from build123d import *

# Parameters (mm, degrees)
SKETCH1_W                       = 203.2
SKETCH1_H                       = 203.2
BOSS_EXTRUDE1_DEPTH             = 6.35
CUT_EXTRUDE1_REACH              = 8.35
SKETCH2_R                       = 31.75
F_1_4_0_25_DIAMETER_HOLE1_D     = 6.35
F_1_4_0_25_DIAMETER_HOLE1_DEPTH = 6.351
CIRPATTERN1_COUNT               = 12
F_10_32_TAPPED_HOLE1_D          = 4.0386
F_10_32_TAPPED_HOLE1_DEPTH      = 6.351
CIRPATTERN2_COUNT               = 6
CUT_EXTRUDE2_REACH              = 8.35


with BuildPart() as part:
    # Sketch1 → Boss-Extrude1 (new body)
    with BuildSketch(Plane(origin=(0, 0, 0), x_dir=(1, 0, 0), z_dir=(0, 1, 0))):
        Rectangle(SKETCH1_W, SKETCH1_H)
    extrude(amount=BOSS_EXTRUDE1_DEPTH)

    # Sketch2 → Cut-Extrude1 (cut, up to next)
    with BuildSketch(Plane(origin=(0, 6.35, 0), x_dir=(1, 0, 0), z_dir=(0, 1, 0)), mode=Mode.PRIVATE) as cut_extrude1_sk1:
        with Locations(Location((0, 0, 0), (0, 0, 270))):  # turned: the seam where the file's is
            Circle(SKETCH2_R)
    cut_extrude1_tool1 = extrude(cut_extrude1_sk1.sketch, amount=-CUT_EXTRUDE1_REACH, mode=Mode.PRIVATE) & part.part
    add(cut_extrude1_tool1.solids().sort_by_distance((0, 6.35, 0))[0], mode=Mode.SUBTRACT)

    # 1/4 (0.25) Diameter Hole1
    with Locations(Plane(origin=(0, 6.35, 0), x_dir=(1, 0, 0), z_dir=(0, 1, 0))):
        with Locations((0, 85.725)):
            f_1_4_0_25_diameter_hole1 = Hole(F_1_4_0_25_DIAMETER_HOLE1_D / 2, depth=F_1_4_0_25_DIAMETER_HOLE1_DEPTH)

    # CirPattern1: 1/4 (0.25) Diameter Hole1 ×12 about axis
    cirpattern1_axis = Axis((0, 0, 0), (0, 1, 0))
    for i in range(1, CIRPATTERN1_COUNT):
        add(f_1_4_0_25_diameter_hole1.rotate(cirpattern1_axis, i * 360 / CIRPATTERN1_COUNT), mode=Mode.SUBTRACT)

    # #10-32 Tapped Hole1
    with Locations(Plane(origin=(0, 6.35, 0), x_dir=(1, 0, 0), z_dir=(0, 1, 0))):
        with Locations((0, 36.5125)):
            f_10_32_tapped_hole1 = Hole(F_10_32_TAPPED_HOLE1_D / 2, depth=F_10_32_TAPPED_HOLE1_DEPTH)

    # CirPattern2: #10-32 Tapped Hole1 ×6 about axis
    cirpattern2_axis = Axis((0, 0, 0), (0, 1, 0))
    for i in range(1, CIRPATTERN2_COUNT):
        add(f_10_32_tapped_hole1.rotate(cirpattern2_axis, i * 360 / CIRPATTERN2_COUNT), mode=Mode.SUBTRACT)

    # Sketch7 → Cut-Extrude2 (cut, up to next)
    with BuildSketch(Plane(origin=(0, 6.35, 0), x_dir=(1, 0, 0), z_dir=(0, 1, 0)), mode=Mode.PRIVATE) as cut_extrude2_sk1:
        with BuildLine():
            ThreePointArc((96.684914721, 45.084916162), (75.434151417, 75.434151417), (45.084916162, 96.684914721))
            ThreePointArc((45.084916162, 96.684914721), (40.865575958, 95.149200478), (42.4012902, 90.929860273))
            ThreePointArc((42.4012902, 90.929860273), (70.944023356, 70.944023356), (90.929860273, 42.4012902))
            ThreePointArc((90.929860273, 42.4012902), (95.149200478, 40.865575958), (96.684914721, 45.084916162))
        make_face()
    cut_extrude2_tool1 = extrude(cut_extrude2_sk1.sketch, amount=-CUT_EXTRUDE2_REACH, mode=Mode.PRIVATE) & part.part
    add(cut_extrude2_tool1.solids().sort_by_distance((71.522214, 6.35, -71.522214))[0], mode=Mode.SUBTRACT)
    # Sketch7 → Cut-Extrude2 (cut, up to next)
    with BuildSketch(Plane(origin=(0, 6.35, 0), x_dir=(1, 0, 0), z_dir=(0, 1, 0)), mode=Mode.PRIVATE) as cut_extrude2_sk2:
        with BuildLine():
            ThreePointArc((45.084916162, -96.684914721), (75.434151417, -75.434151417), (96.684914721, -45.084916162))
            ThreePointArc((96.684914721, -45.084916162), (95.149200478, -40.865575958), (90.929860273, -42.4012902))
            ThreePointArc((90.929860273, -42.4012902), (70.944023356, -70.944023356), (42.4012902, -90.929860273))
            ThreePointArc((42.4012902, -90.929860273), (40.865575958, -95.149200478), (45.084916162, -96.684914721))
        make_face()
    cut_extrude2_tool2 = extrude(cut_extrude2_sk2.sketch, amount=-CUT_EXTRUDE2_REACH, mode=Mode.PRIVATE) & part.part
    add(cut_extrude2_tool2.solids().sort_by_distance((71.522214, 6.35, 71.522214))[0], mode=Mode.SUBTRACT)
    # Sketch7 → Cut-Extrude2 (cut, up to next)
    with BuildSketch(Plane(origin=(0, 6.35, 0), x_dir=(1, 0, 0), z_dir=(0, 1, 0)), mode=Mode.PRIVATE) as cut_extrude2_sk3:
        with BuildLine():
            ThreePointArc((-96.684914721, -45.084916162), (-75.434151417, -75.434151417), (-45.084916162, -96.684914721))
            ThreePointArc((-45.084916162, -96.684914721), (-40.865575958, -95.149200478), (-42.4012902, -90.929860273))
            ThreePointArc((-42.4012902, -90.929860273), (-70.944023356, -70.944023356), (-90.929860273, -42.4012902))
            ThreePointArc((-90.929860273, -42.4012902), (-95.149200478, -40.865575958), (-96.684914721, -45.084916162))
        make_face()
    cut_extrude2_tool3 = extrude(cut_extrude2_sk3.sketch, amount=-CUT_EXTRUDE2_REACH, mode=Mode.PRIVATE) & part.part
    add(cut_extrude2_tool3.solids().sort_by_distance((-71.522214, 6.35, 71.522214))[0], mode=Mode.SUBTRACT)
    # Sketch7 → Cut-Extrude2 (cut, up to next)
    with BuildSketch(Plane(origin=(0, 6.35, 0), x_dir=(1, 0, 0), z_dir=(0, 1, 0)), mode=Mode.PRIVATE) as cut_extrude2_sk4:
        with BuildLine():
            ThreePointArc((-45.084916162, 96.684914721), (-75.434151417, 75.434151417), (-96.684914721, 45.084916162))
            ThreePointArc((-96.684914721, 45.084916162), (-95.149200478, 40.865575958), (-90.929860273, 42.4012902))
            ThreePointArc((-90.929860273, 42.4012902), (-70.944023356, 70.944023356), (-42.4012902, 90.929860273))
            ThreePointArc((-42.4012902, 90.929860273), (-40.865575958, 95.149200478), (-45.084916162, 96.684914721))
        make_face()
    cut_extrude2_tool4 = extrude(cut_extrude2_sk4.sketch, amount=-CUT_EXTRUDE2_REACH, mode=Mode.PRIVATE) & part.part
    add(cut_extrude2_tool4.solids().sort_by_distance((-71.522214, 6.35, -71.522214))[0], mode=Mode.SUBTRACT)


solid = part.part
The model under review builds one solid part; all positions refer to its coordinate system, in mm. A direction names the side the tool comes from. Round coordinates to 2 decimals unless told otherwise and drop trailing zeros. Order: outer loops, then holes, each group sorted by start corner. A loop starts at its lowest first (then second) coordinate and runs counter-clockwise, first axis right, second up. Notation, with made-up numbers: (11.5, 87) -> (65.5, 87) arc R10 cw to (65.5, 97) -> close; hole circle Ø4 at (4.25, 36.5). An arc over 180 degrees is marked (long way). Write item = value, one per line. Start each with the question number.
Item 1: For faces 1 (the face through (101.6, 3, 1)), 2 (the face through (75.802, 3.219, -75.065)), list the 3-axis set-ups (+Z, -Z, +X, -X, +Y, -Y) from which the entire face can be reached by the end or side of a thin tool; tool diameter is ignored.
Item 2: Consider section D-D on x = -27. Write out the cut boundary in (y, z), plus the area to 3 significant figures.
Item 3: Consider section B-B on x = 62.5. Write out the cut boundary in (y, z).
Item 4: Consider section A-A on z = 0. Write out the cut boundary in (x, y).
Item 5: For line 1 along X through (y, z) = (4, 0); line 2 along X through (y, z) = (1, -2); line 3 along Z through (x, y) = (-84.5, 5.75), list the stretches that pass through material, from the lowest coordinate up.
Item 6: Mouldability with a two-part tool opening along Z and no side actions: class faces 3 (the face through (-1, 3, -101.6)), 4 (the face through (-45.96, 3.13, 74.93)), 5 (the face through (-101.6, 3, 1)) as released by +Z, released by -Z, zero draft, split by the parting line, or undercut.
Item 7: Consider section C-C on z = -60. Write out the cut boundary in (x, y), plus the area to 3 significant figures.
Item 8: Clearance check with flat-ended pins moving along their axes: pin 1 Ø3.5 at (x, z) = (-31.62, 18.26) entering from +Y; pin 2 Ø5.5 at (x, z) = (31.62, 18.26) entering from +Y. State where each tip first meets the part, or that it passes through.
Conclusion:
q1.face_1 = +Z, -Z, +X, +Y, -Y
q1.face_2 = +Y, -Y
q2.outline = (0, -101.6) -> (6.35, -101.6) -> (6.35, -16.71) -> (0, -16.71) -> close; (0, 16.71) -> (6.35, 16.71) -> (6.35, 101.6) -> (0, 101.6) -> close
q2.area = 1,080 mm2
q3.outline = (0, -101.6) -> (6.35, -101.6) -> (6.35, -86.45) -> (0, -86.45) -> close; (0, -78.48) -> (6.35, -78.48) -> (6.35, 78.48) -> (0, 78.48) -> close; (0, 86.45) -> (6.35, 86.45) -> (6.35, 101.6) -> (0, 101.6) -> close
q4.outline = (-101.6, 0) -> (-88.9, 0) -> (-88.9, 6.35) -> (-101.6, 6.35) -> close; (-82.55, 0) -> (-31.75, 0) -> (-31.75, 6.35) -> (-82.55, 6.35) -> close; (31.75, 0) -> (82.55, 0) -> (82.55, 6.35) -> (31.75, 6.35) -> close; (88.9, 0) -> (101.6, 0) -> (101.6, 6.35) -> (88.9, 6.35) -> close
q5.line_1 = -101.6 to -88.9, -82.55 to -31.75, 31.75 to 82.55, 88.9 to 101.6
q5.line_2 = -101.6 to -88.19, -83.26 to -31.69, 31.69 to 83.26, 88.19 to 101.6
q5.line_3 = -101.6 to -65.12, -54.09 to -2.93, 2.93 to 54.09, 65.12 to 101.6
q6.face_3 = released by -Z
q6.face_4 = undercut
q6.face_5 = zero draft
q7.outline = (-101.6, 0) -> (-88.21, 0) -> (-88.21, 6.35) -> (-101.6, 6.35) -> close; (-80.41, 0) -> (80.41, 0) -> (80.41, 6.35) -> (-80.41, 6.35) -> close; (88.21, 0) -> (101.6, 0) -> (101.6, 6.35) -> (88.21, 6.35) -> close
q7.area = 1,190 mm2
q8.pin_1 = through
q8.pin_2 = 6.35
